Source: three-view drawing plus pictorial views. Frame: mm from the lowest corner of the part. A direction names the side the tool comes from. Give positions to 0.01 mm unless a question says otherwise; leave off trailing zeros. Loops run counter-clockwise (first coordinate to the right, second up) from the corner with the lowest first, then second, coordinate; pieces in that order, holes last. Notation, with made-up numbers: (68.5, -23) - (82.5, -23) arc R23 ccw to (82.5, -12) - close; hole circle Ø1 at (-25.75, 47.5). An arc over 180 degrees is marked (long way). Answer as a JSON object with one key per item and string values. Group by question number.
(1) Section query C-C (z = 4.75). Return loops of the section in (x, y).
(2) Pin query (flat end, axial travel): P1, Ø7, axis at x = 10, y = 25, coming from the +Z side. Return the tip coordinate at first contact, or that it passes through.
(3) Section query A-A (x = 10). Return loops of the section in (y, z), plus the area to 3 significant figures.
(4) Material intervals for L1, parallel to Y at x = 10, z = 0.65; L2, parallel to Y at x = 10, z = 5; L3, parallel to Z at x = 18, y = 2, sorted ascending.
(5) Section query B-B (y = 15). Return loops of the section in (x, z).
(6) Section query D-D (x = 5.25). Return loops of the section in (y, z), plus the area to 3 significant figures.
(7) Access query for the marked faces 1 and 2. Directions: +Z, -Z, +X, -X, +Y, -Y. A direction counts if a zero-diameter tool reaches every point of the face in a straight line with its end or side. Return the directions, or none.
(8) Mould query, pull axis Y, two halves, no side actions, for the marked faces 3, 4 and 5. Classes: +Y half, -Y half, draft (parallel to the pull), parting line (faces both ways), or undercut.
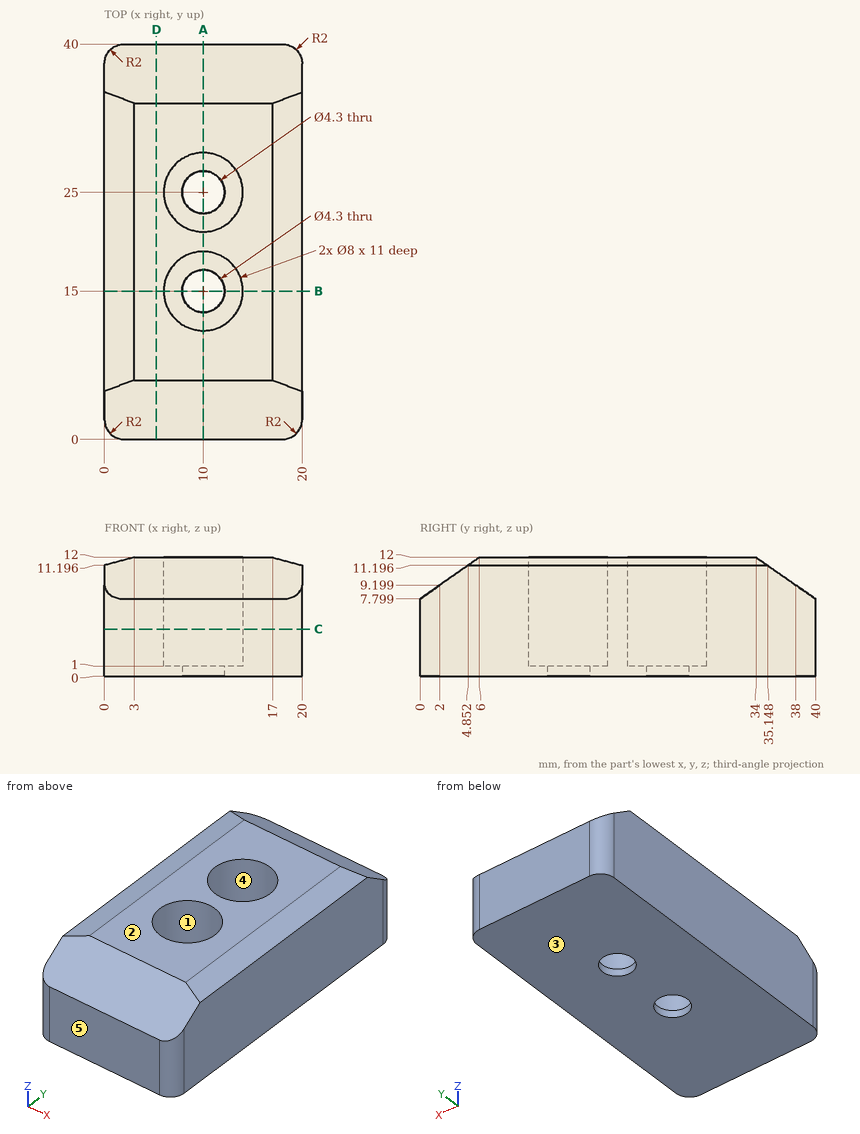
Recorded:
{
 "1": {"outline": "(0, 2) arc R2 ccw to (2, 0) - (18, 0) arc R2 ccw to (20, 2) - (20, 38) arc R2 ccw to (18, 40) - (2, 40) arc R2 ccw to (0, 38) - close; hole circle Ø8 at (10, 15); hole circle Ø8 at (10, 25)"},
 "2": {"P1": "stops at z = 1"},
 "3": {"outline": "(0, 0) - (12.85, 0) - (12.85, 1) - (11, 1) - (11, 12) - (6, 12) - (0, 7.8) - close; (17.15, 0) - (22.85, 0) - (22.85, 1) - (21, 1) - (21, 12) - (19, 12) - (19, 1) - (17.15, 1) - close; (27.15, 0) - (40, 0) - (40, 7.8) - (34, 12) - (29, 12) - (29, 1) - (27.15, 1) - close", "area": "270 mm^2"},
 "4": {"L1": "y = 0 to 12.85, 17.15 to 22.85, 27.15 to 40", "L2": "y = 0 to 11, 19 to 21, 29 to 40", "L3": "z = 0 to 9.2"},
 "5": {"outline": "(0, 0) - (7.85, 0) - (7.85, 1) - (6, 1) - (6, 12) - (3, 12) - (0, 11.2) - close; (12.15, 0) - (20, 0) - (20, 11.2) - (17, 12) - (14, 12) - (14, 1) - (12.15, 1) - close"},
 "6": {"outline": "(0, 0) - (40, 0) - (40, 7.8) - (34, 12) - (6, 12) - (0, 7.8) - close", "area": "455 mm^2"},
 "7": {"face 1": "+Z", "face 2": "+Z, +X, -X, +Y, -Y"},
 "8": {"face 3": "draft", "face 4": "undercut", "face 5": "-Y half"}
}
